from build123d import *

# Parameters (mm, degrees)
SKETCH1_W           = 25.4
SKETCH1_H           = 25.4
SKETCH1_W_2         = 22.2504
SKETCH1_H_2         = 22.2504
BOSS_EXTRUDE1_DEPTH = 609.6
FILLET1_R           = 3.175


with BuildPart() as part:
    # Sketch1 → Boss-Extrude1 (new body, symmetric)
    with BuildSketch(Plane.XY):
        Rectangle(SKETCH1_W, SKETCH1_H)
        Rectangle(SKETCH1_W_2, SKETCH1_H_2, mode=Mode.SUBTRACT)
    extrude(amount=BOSS_EXTRUDE1_DEPTH, both=True)

    # Fillet1
    fillet1_edges = [part.edges().sort_by_distance(p)[0] for p in [
        (11.1252, -11.1252, 0),
        (11.1252, 11.1252, 0),
        (-11.1252, 11.1252, 0),
        (-11.1252, -11.1252, 0),
        (12.7, -12.7, 0),
        (-12.7, -12.7, 0),
        (-12.7, 12.7, 0),
        (12.7, 12.7, 0),
    ]]
    fillet(fillet1_edges, radius=FILLET1_R)


solid = part.part
Here's how the part is built. I have some questions about the finished solid (model axes, mm). Give positions to 0.01 mm unless a question says otherwise; leave off trailing zeros. Order: outer loops, then holes, each group sorted by start corner. A loop starts at its lowest first (then second) coordinate and runs counter-clockwise, first axis right, second up. Notation, with made-up numbers: (-31, 44) -> (14, 44) arc R25 cw to (14, 71) -> close; hole circle Ø11 at (23.5, 59.5). An arc over 180 degrees is marked (long way). One line per item, written item: value. Start each with the question number.
1. Imagine slicing it at A-A, the plane y = -2.5. List the corners of the cut face in (x, z) for me.
2. Imagine slicing it at C-C, the plane z = 48. List the corners of the cut face in (x, y) for me (3 decimals), plus the area to 3 significant figures.
3. I need wall thicknesses on probe 1 along X at (y, z) = (-2, -170.5); probe 2 along Y at (x, z) = (-9, -31). Which ranges of each line are inside material? Lowest first, please. Write a range as from..to.
Values follow:
1. outline: (-12.7, -609.6) -> (-11.13, -609.6) -> (-11.13, 609.6) -> (-12.7, 609.6) -> close; (11.13, -609.6) -> (12.7, -609.6) -> (12.7, 609.6) -> (11.13, 609.6) -> close
2. outline: (-12.7, -9.525) arc R3.175 ccw to (-9.525, -12.7) -> (9.525, -12.7) arc R3.175 ccw to (12.7, -9.525) -> (12.7, 9.525) arc R3.175 ccw to (9.525, 12.7) -> (-9.525, 12.7) arc R3.175 ccw to (-12.7, 9.525) -> close; hole (-11.125, -7.95) arc R3.175 ccw to (-7.95, -11.125) -> (7.95, -11.125) arc R3.175 ccw to (11.125, -7.95) -> (11.125, 7.95) arc R3.175 ccw to (7.95, 11.125) -> (-7.95, 11.125) arc R3.175 ccw to (-11.125, 7.95) -> close
2. area: 150 mm2
3. probe 1: x = -12.7..-11.13, 11.13..12.7
3. probe 2: y = -12.7..-10.95, 10.95..12.7
